Check sheet for the modelled part. Datum: model origin and axes. Units: mm. A direction names the side the tool comes from. Give positions to 0.01 mm unless a question says otherwise; leave off trailing zeros. Order: outer loops, then holes, each group sorted by start corner. A loop starts at its lowest first (then second) coordinate and runs counter-clockwise, first axis right, second up. Notation, with made-up numbers: (26.5, 1.5) -> (82.5, 1.5) arc R20 ccw to (82.5, 12.5) -> close; hole circle Ø4 at (22, -26). An arc over 180 degrees is marked (long way). Write each question's results on one line, items separated by ' | '.
from build123d import *

# Parameters (mm, degrees)
BOSS_EXTRUDE2_DEPTH = 38.1
SKETCH1_W           = 25.35
SKETCH1_H           = 29.67
BOSS_EXTRUDE3_DEPTH = 3.81
SKETCH3_W           = 3
SKETCH3_H           = 7.62
CUT_EXTRUDE1_DEPTH  = 4.81
SKETCH4_W           = 7.62
SKETCH4_H           = 30.1
CUT_EXTRUDE2_DEPTH  = 4.81
SKETCH5_R           = 1.5
CUT_EXTRUDE3_DEPTH  = 4.81
SKETCH6_R           = 1.45
CUT_EXTRUDE4_DEPTH  = 24.844
FILLET1_R           = 4
FILLET4_R           = 2.54
FILLET2_R           = 1.016
FILLET3_R           = 1.27
FILLET5_R           = 1.016
CUT_EXTRUDE5_DEPTH  = 1.27
CUT_EXTRUDE6_DEPTH  = 1.27


with BuildPart() as part:
    # Sketch2 → Boss-Extrude2 (new body)
    with BuildSketch(Plane(origin=(0, 0, 0), x_dir=(1, 0, 0), z_dir=(0, 1, 0))):
        Polygon((-9.5, -11.43), (9.5, -11.43), (9.5, -5.08), (12.04, -5.08), (12.04, -14.43), (-13.31, -14.43), (-13.31, 15.24), (12.04, 15.24), (12.04, 7.62), (9.5, 7.62), (9.5, 11.43), (-9.5, 11.43), align=None)
    extrude(amount=BOSS_EXTRUDE2_DEPTH)

    # Sketch1 → Boss-Extrude3 (add)
    with BuildSketch(Plane(origin=(0, 0, 0), x_dir=(1, 0, 0), z_dir=(0, 1, 0))):
        with Locations((-0.635, 0.405)):
            Rectangle(SKETCH1_W, SKETCH1_H)
    extrude(amount=-BOSS_EXTRUDE3_DEPTH)

    # Sketch3 → Cut-Extrude1 (cut, through all)
    with BuildSketch(Plane(origin=(0, 0, 0), x_dir=(1, 0, 0), z_dir=(0, 1, 0))):
        with Locations((-0.38, 0)):
            Rectangle(SKETCH3_W, SKETCH3_H)
    extrude(amount=-CUT_EXTRUDE1_DEPTH, mode=Mode.SUBTRACT)

    # Sketch4 → Cut-Extrude2 (cut, through all)
    with BuildSketch(Plane(origin=(-9.5, 0, 0), x_dir=(0, 0, -1), z_dir=(1, 0, 0))):
        with Locations((0, 23.05)):
            Rectangle(SKETCH4_W, SKETCH4_H)
    extrude(amount=-CUT_EXTRUDE2_DEPTH, mode=Mode.SUBTRACT)

    # Sketch5 → Cut-Extrude3 (cut, through all)
    with BuildSketch(Plane(origin=(-9.5, 0, 0), x_dir=(0, 0, -1), z_dir=(1, 0, 0))):
        with Locations((-9.1700096, 31)):
            Circle(SKETCH5_R)
        with Locations((8.2299904, 31)):
            Circle(SKETCH5_R)
    extrude(amount=-CUT_EXTRUDE3_DEPTH, mode=Mode.SUBTRACT)

    # Sketch6 → Cut-Extrude4 (cut)
    with BuildSketch(Plane.XY.offset(14.43)):
        with Locations((-11.405, 19.05)):
            Circle(SKETCH6_R)
        with Locations((-3.81, -1.905)):
            Circle(SKETCH6_R)
    extrude(amount=-CUT_EXTRUDE4_DEPTH, mode=Mode.SUBTRACT)

    # Fillet1
    fillet1_edges = [part.edges().sort_by_distance(p)[0] for p in [
        (0, 0, -11.43),
        (0, 0, 11.43),
    ]]
    fillet(fillet1_edges, radius=FILLET1_R)


with BuildPart() as body_2:
    # Mirror1: mirrored copy
    add(part.part.mirror(Plane.XY))

    # Fillet4
    fillet4_edges = [body_2.edges().sort_by_distance(p)[0] for p in [
        (-11.405, 8, -3.81),
        (-11.405, 8, 3.81),
    ]]
    fillet(fillet4_edges, radius=FILLET4_R)

    # Fillet2
    fillet2_edges = [body_2.edges().sort_by_distance(p)[0] for p in [
        (-13.31, 17.145, 15.24),
        (12.04, 17.145, 15.24),
        (12.04, -3.81, 0.405),
        (-13.31, -3.81, 0.405),
        (-0.635, -3.81, 15.24),
        (12.04, 38.1, 11.43),
        (-0.635, 38.1, 15.24),
        (-13.31, 38.1, 9.525),
        (-13.31, 38.1, -9.12),
        (-11.405, 38.1, -3.81),
        (-11.405, 38.1, 3.81),
    ]]
    fillet(fillet2_edges, radius=FILLET2_R)

    # Fillet3
    fillet3_edges = [body_2.edges().sort_by_distance(p)[0] for p in [
        (-1.88, 0, 0),
        (-0.38, 0, -3.81),
        (1.12, 0, 0),
        (-0.38, 0, 3.81),
    ]]
    fillet(fillet3_edges, radius=FILLET3_R)

    # Fillet5
    fillet5_edges = [body_2.edges().sort_by_distance(p)[0] for p in [
        (12.04, 38.1, -9.755),
        (10.77, 38.1, -5.08),
    ]]
    fillet(fillet5_edges, radius=FILLET5_R)


with BuildPart() as body_2_2:
    # Mirror3: mirrored copy
    add(body_2.part.mirror(Plane.ZY.offset(15.85)))

    # Sketch8 → Cut-Extrude6 (cut)
    with BuildSketch(Plane(origin=(0, 0, 0), x_dir=(1, 0, 0), z_dir=(0, 1, 0))):
        Polygon((-35.125709402, -4.085355142), (-35.125709402, -4.750205569), (-37.310217949, -4.750205569), (-37.310217949, -5.699991894), (-37.975068376, -5.699991894), (-37.975068376, -4.750205569), (-42.724, -4.750205569), (-42.724, -4.085355142), (-37.975068376, -4.085355142), (-37.975068376, -3.135568817), (-37.310217949, -3.135568817), (-37.310217949, -4.085355142), align=None)
        with BuildLine():
            Line((-35.315666667, 2.658127764), (-35.315666667, 1.175570673))
            add(Edge.make_bspline(
                [(-35.315666667, 1.175570673), (-35.31599599, 1.076635284), (-35.316628328, 0.886668378), (-35.320154193, 0.614521623), (-35.330259913, 0.367237601), (-35.338956414, 0.144945608), (-35.354814357, -0.052350279), (-35.36997106, -0.225255044), (-35.389811975, -0.372972337), (-35.408238454, -0.462392723), (-35.416581464, -0.502879848)],
                knots=[0, 0, 0, 0, 0.000296812, 0.000569912, 0.000816423, 0.001039272, 0.001237207, 0.001410128, 0.001559979, 0.001683965, 0.001683965, 0.001683965, 0.001683965], degree=3))
            add(Edge.make_bspline(
                [(-35.416581464, -0.502879848), (-35.429971598, -0.557081491), (-35.456466218, -0.664328507), (-35.512494413, -0.81872563), (-35.577224639, -0.965915382), (-35.653842803, -1.105345402), (-35.741012521, -1.237028627), (-35.839243094, -1.360767889), (-35.949034771, -1.475855736), (-36.067583937, -1.583177714), (-36.195924968, -1.680461633), (-36.332188282, -1.764648136), (-36.475521634, -1.836736616), (-36.626424162, -1.894287018), (-36.783620234, -1.940584552), (-36.948482467, -1.973239748), (-37.120273858, -1.992820602), (-37.237448007, -1.99481431), (-37.296861579, -1.995825227)],
                knots=[0, 0, 0, 0, 0.000167388, 0.000331205, 0.000491982, 0.000649388, 0.000807854, 0.000965226, 0.001122688, 0.00128451, 0.00144449, 0.001605103, 0.001764387, 0.001925062, 0.002088959, 0.002255437, 0.002428663, 0.002606847, 0.002606847, 0.002606847, 0.002606847], degree=3))
            add(Edge.make_bspline(
                [(-37.296861579, -1.995825227), (-37.395572664, -1.992715929), (-37.588183557, -1.986648882), (-37.867710836, -1.930079619), (-38.128467354, -1.83742344), (-38.370090229, -1.709723959), (-38.587996871, -1.547178937), (-38.778744039, -1.351836783), (-38.939838712, -1.124695094), (-39.050363857, -0.91224832), (-39.121480472, -0.724494941), (-39.171769577, -0.569470973), (-39.209969011, -0.400237622), (-39.244686959, -0.219222799), (-39.271179543, -0.025028326), (-39.289994312, 0.181954737), (-39.302092352, 0.402244067), (-39.303859928, 0.553246562), (-39.304769231, 0.630927577)],
                knots=[0, 0, 0, 0, 0.000295861, 0.000577301, 0.000851427, 0.001123618, 0.001394011, 0.001663719, 0.001939227, 0.00222663, 0.002379313, 0.002541237, 0.002715098, 0.00289934, 0.003094106, 0.003302766, 0.003522724, 0.003755761, 0.003755761, 0.003755761, 0.003755761], degree=3))
            Line((-39.304769231, 0.630927577), (-42.724, -2.09080386))
            Line((-42.724, -2.09080386), (-42.724, -1.268645072))
            Line((-42.724, -1.268645072), (-39.304769231, 1.453086364))
            Line((-39.304769231, 1.453086364), (-39.304769231, 1.993277337))
            Line((-39.304769231, 1.993277337), (-42.724, 1.993277337))
            Line((-42.724, 1.993277337), (-42.724, 2.658127764))
            Line((-42.724, 2.658127764), (-35.315666667, 2.658127764))
        make_face()
        with BuildLine():
            Line((-36.075495726, 1.993277337), (-38.544940171, 1.993277337))
            Line((-38.544940171, 1.993277337), (-38.555328459, 0.636863742))
            add(Edge.make_bspline(
                [(-38.555328459, 0.636863742), (-38.555356476, 0.573532993), (-38.555410782, 0.450779964), (-38.546957292, 0.27319022), (-38.537340592, 0.107835996), (-38.522631175, -0.044650303), (-38.503674054, -0.184336572), (-38.479961405, -0.31115373), (-38.452333452, -0.425306376), (-38.409577922, -0.55844757), (-38.341800903, -0.707074645), (-38.243358644, -0.86880077), (-38.118738571, -1.006056387), (-37.978502281, -1.124397331), (-37.821144229, -1.215549999), (-37.653648946, -1.281893149), (-37.477462473, -1.323527172), (-37.356448737, -1.328476869), (-37.295377537, -1.3309748)],
                knots=[0, 0, 0, 0, 0.000189963, 0.000368203, 0.000533258, 0.000686833, 0.000827661, 0.00095602, 0.001073718, 0.001179783, 0.001375069, 0.001562422, 0.001745315, 0.001928677, 0.002110918, 0.002288116, 0.002467759, 0.002650784, 0.002650784, 0.002650784, 0.002650784], degree=3))
            add(Edge.make_bspline(
                [(-37.295377537, -1.3309748), (-37.235784101, -1.328469191), (-37.117691657, -1.323503988), (-36.945281883, -1.281812481), (-36.781395026, -1.214486794), (-36.629154879, -1.120080599), (-36.489810496, -1.006005192), (-36.372231955, -0.870523684), (-36.27376678, -0.720459089), (-36.211303642, -0.580102451), (-36.172931546, -0.454736188), (-36.145962748, -0.345871562), (-36.124112719, -0.222396299), (-36.107124734, -0.084606312), (-36.091837488, 0.067249114), (-36.081925643, 0.233585788), (-36.075934923, 0.414211629), (-36.075645532, 0.539406498), (-36.075495726, 0.604214837)],
                knots=[0, 0, 0, 0, 0.000178585, 0.00035389, 0.000528894, 0.000708076, 0.000889348, 0.001067068, 0.001244067, 0.001426091, 0.001525599, 0.001637179, 0.00176235, 0.00190151, 0.002053608, 0.002220145, 0.002401295, 0.00259571, 0.00259571, 0.00259571, 0.00259571], degree=3))
            Line((-36.075495726, 0.604214837), (-36.075495726, 1.993277337))
        make_face(mode=Mode.SUBTRACT)
    extrude(amount=-CUT_EXTRUDE6_DEPTH, mode=Mode.SUBTRACT)


with BuildPart() as body_2_1:
    add(body_2.part)

    # Sketch7 → Cut-Extrude5 (cut)
    with BuildSketch(Plane(origin=(0, 0, 0), x_dir=(1, 0, 0), z_dir=(0, 1, 0))):
        Polygon((4.129986879, -2.992887734), (4.129986879, -2.328037307), (10.778491153, -2.328037307), (10.778491153, 0.521321667), (11.538320213, 0.521321667), (11.538320213, -2.992887734), align=None)
        Polygon((3.940029614, 2.230937052), (3.940029614, 2.895787479), (6.124538161, 2.895787479), (6.124538161, 3.845573804), (6.789388589, 3.845573804), (6.789388589, 2.895787479), (11.538320213, 2.895787479), (11.538320213, 2.230937052), (6.789388589, 2.230937052), (6.789388589, 1.281150727), (6.124538161, 1.281150727), (6.124538161, 2.230937052), align=None)
    extrude(amount=-CUT_EXTRUDE5_DEPTH, mode=Mode.SUBTRACT)


solid = body_2_2.part
1. Material ranges on probe 1 along X at (y, z) = (21, 9); probe 2 along Z at (x, y) = (-27, 4); probe 3 along Z at (x, y) = (-20, 20), recorded low to high. Write a range as from..to.
Verdict:
probe 1: x = -43.74..-41.2, -22.2..-18.39 | probe 2: z = -14.43..-11.43, 11.43..15.24 | probe 3: z = 10.41..15.24
2. Gauge pin test, flat ends, axial feed: pin 1 Ø1 at (x, z) = (-37, 0.5) entering from +Y; pin 2 Ø2 at (y, z) = (17.5, 1) entering from +X. Record the tip position at first contact, or that the pin passes through.
Verdict:
pin 1: stops at y = 0 | pin 2: passes through
3. Section check D-D on x = -27.89. Record the cut outline in (y, z) (3 decimals), then the cut area to 3 significant figures.
Verdict:
outline: (-3.81, -14.43) -> (-3.355, -14.43) -> (-3.355, 10.414) -> (-0.455, 10.414) -> (-0.455, -14.43) -> (38.1, -14.43) -> (38.1, -11.43) -> (4, -11.43) arc R4 cw to (0, -7.43) -> (0, 7.43) arc R4 cw to (4, 11.43) -> (38.1, 11.43) -> (38.1, 14.224) arc R1.016 ccw to (37.084, 15.24) -> (-2.794, 15.24) arc R1.016 ccw to (-3.81, 14.224) -> close | area: 307 mm^2
4. Section check A-A on y = 31. Record the cut outline in (x, z), then the cut area to 3 significant figures.
Verdict:
outline: (-43.74, -14.43) -> (-18.39, -14.43) -> (-18.39, -10.67) -> (-22.2, -10.67) -> (-22.2, -11.43) -> (-41.2, -11.43) -> (-41.2, -5.08) -> (-43.74, -5.08) -> close; (-43.74, 7.62) -> (-41.2, 7.62) -> (-41.2, 11.43) -> (-22.2, 11.43) -> (-22.2, 9.73) -> (-18.39, 9.73) -> (-18.39, 14.22) arc R1.02 ccw to (-19.41, 15.24) -> (-42.72, 15.24) arc R1.02 ccw to (-43.74, 14.22) -> close; (-22.2, -7.67) -> (-18.39, -7.67) -> (-18.39, -3.81) -> (-22.2, -3.81) -> close; (-22.2, 3.81) -> (-18.39, 3.81) -> (-18.39, 6.73) -> (-22.2, 6.73) -> close | area: 233 mm^2
5. Section check B-B on y = 19.05. Record the cut outline in (x, z) (3 decimals), then the cut area to 3 significant figures.
Verdict:
outline: (-43.74, -14.43) -> (-21.745, -14.43) -> (-21.745, -3.81) -> (-22.2, -3.81) -> (-22.2, -11.43) -> (-41.2, -11.43) -> (-41.2, -5.08) -> (-43.74, -5.08) -> close; (-43.74, 7.62) -> (-41.2, 7.62) -> (-41.2, 11.43) -> (-22.2, 11.43) -> (-22.2, 3.81) -> (-21.745, 3.81) -> (-21.745, 10.414) -> (-18.845, 10.414) -> (-18.845, 3.81) -> (-18.39, 3.81) -> (-18.39, 14.224) arc R1.016 ccw to (-19.406, 15.24) -> (-42.724, 15.24) arc R1.016 ccw to (-43.74, 14.224) -> close; (-18.845, -14.43) -> (-18.39, -14.43) -> (-18.39, -3.81) -> (-18.845, -3.81) -> close | area: 206 mm^2
6. Section check C-C on z = -10. Record the cut outline in (x, y) (3 decimals).
Verdict:
outline: (-43.74, -2.794) arc R1.016 ccw to (-42.724, -3.81) -> (-19.406, -3.81) arc R1.016 ccw to (-18.39, -2.794) -> (-18.39, 29.751) -> (-22.2, 29.751) -> (-22.2, 0.935) -> (-41.2, 0.935) -> (-41.2, 38.1) -> (-42.724, 38.1) arc R1.016 ccw to (-43.74, 37.084) -> close; (-22.2, 32.249) -> (-18.39, 32.249) -> (-18.39, 37.084) arc R1.016 ccw to (-19.406, 38.1) -> (-22.2, 38.1) -> close; hole circle Ø2.9 at (-27.89, -1.905); hole circle Ø2.9 at (-20.295, 19.05)
7. Access from +Z, -Z, +X, -X, +Y, -Y to the whole of each face (thin tool, end or side, straight path). Record for faces 1 (the cylindrical face through (-20.268, 8.764, -3.086)), 2 (the flat face through (-20, 19, 10.414)), 3 (the flat face through (-41.04, -0.63, -0.07)).
Verdict:
face 1: +X, -X, +Y | face 2: -Z | face 3: +Y
8. Mould release check, pull along X, two halves, no side actions. Record for faces 4 (the flat face through (-41.2, 19, 9)), 5 (the flat face through (-31, 38.1, -12)), 6 (the cylindrical face through (-18.68, -3.504, 0.098)): +X half, -X half, draft (parallel to the pull), parting line (faces both ways), or undercut.
Verdict:
face 4: undercut | face 5: draft | face 6: +X half
